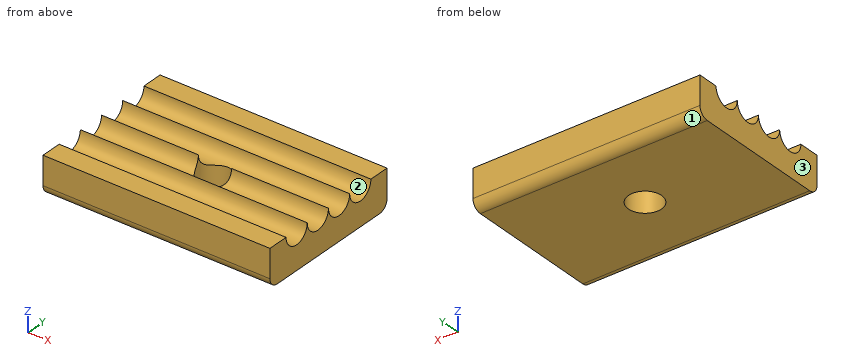
from build123d import *

# Parameters (mm, degrees)
SKETCH2_W           = 24
SKETCH2_H           = 16
BOSS_EXTRUDE1_DEPTH = 4
SKETCH3_R           = 1.75
CUT_EXTRUDE1_DEPTH  = 5
FILLET1_R           = 1
CUT_EXTRUDE2_DEPTH  = 29


with BuildPart() as part:
    # Sketch2 → Boss-Extrude1 (new body)
    with BuildSketch(Plane.XY):
        with Locations((6.957345972, -4)):
            Rectangle(SKETCH2_W, SKETCH2_H)
    extrude(amount=BOSS_EXTRUDE1_DEPTH)

    # Sketch3 → Cut-Extrude1 (cut)
    with BuildSketch(Plane.XY.offset(4)):
        with Locations((6.957345972, -4)):
            Circle(SKETCH3_R)
    extrude(amount=-CUT_EXTRUDE1_DEPTH, mode=Mode.SUBTRACT)

    # Fillet1
    fillet1_edges = [part.edges().sort_by_distance(p)[0] for p in [
        (6.957345972, 4, 0),
        (6.957345972, -12, 0),
    ]]
    fillet(fillet1_edges, radius=FILLET1_R)

    # Sketch4 → Cut-Extrude2 (cut)
    with BuildSketch(Plane.ZY.offset(5.042654028)):
        with BuildLine():
            ThreePointArc((5.45, -8.35), (5.025304833, -7.324695167), (4, -6.9))
            Line((4, -6.9), (4, -9.8))
            ThreePointArc((4, -9.8), (5.025304833, -9.375304833), (5.45, -8.35))
        make_face()
        with BuildLine():
            Line((4, -9.8), (4, -6.9))
            ThreePointArc((4, -6.9), (2.55, -8.35), (4, -9.8))
        make_face()
        with BuildLine():
            ThreePointArc((4, -6.9), (5.025304833, -6.475304833), (5.45, -5.45))
            ThreePointArc((5.45, -5.45), (5.025304832, -4.424695167), (3.999999999, -4))
            Line((4, -4), (4, -6.9))
        make_face()
        with BuildLine():
            Line((4, -6.9), (4, -4))
            ThreePointArc((3.999999999, -4), (2.55, -5.450000001), (4, -6.9))
        make_face()
        with BuildLine():
            ThreePointArc((4, -1.1), (2.55, -2.549999999), (3.999999999, -4))
            Line((4, -4), (4, -1.1))
        make_face()
        with BuildLine():
            Line((4, -1.1), (4, -4))
            ThreePointArc((3.999999999, -4), (5.025304832, -3.575304833), (5.45, -2.55))
            ThreePointArc((5.45, -2.55), (5.025304833, -1.524695167), (4, -1.1))
        make_face()
        with BuildLine():
            ThreePointArc((4, 1.8), (2.55, 0.35), (4, -1.1))
            Line((4, -1.1), (4, 1.8))
        make_face()
        with BuildLine():
            Line((4, 1.8), (4, -1.1))
            ThreePointArc((4, -1.1), (5.025304833, -0.675304833), (5.45, 0.35))
            ThreePointArc((5.45, 0.35), (5.025304833, 1.375304833), (4, 1.8))
        make_face()
    extrude(amount=-CUT_EXTRUDE2_DEPTH, mode=Mode.SUBTRACT)


solid = part.part
Build history of the part. All positions in model axes, mm. Face numbers are marked on the shaded views. Coordinates: 2 decimals unless noted, no trailing zeros. Order: outer loops, then holes, each group sorted by start corner. A loop starts at its lowest first (then second) coordinate and runs counter-clockwise, first axis right, second up. Notation, with made-up numbers: (82, 5.25) - (113, 5.25) arc R23 cw to (113, 44.25) - close; hole circle Ø7 at (36.5, -13.75). An arc over 180 degrees is marked (long way). Write item = value, one per line. Start each with the question number.
1) Flat gauge pin, fed straight in: pin 1 Ø3 at (x, y) = (6.96, -4) entering from +Z. Where does the tip first touch, or does it go through?
2) Saw through at C-C on y = -5.45. Write the cut outline in (x, z), then the cut area to 3 significant figures.
3) Saw through at B-B on x = 2. Write the cut outline in (y, z).
4) Wall check: line 1 along X through (y, z) = (-4, 0.9); line 2 along Y through (x, z) = (15.5, 3.5); line 3 along Y through (x, z) = (-0.75, 2.7). Give the ranges that are in metal, low to high. Write a range as from..to.
5) Saw through at A-A on z = 3. Write the cut outline in (x, y).
6) Two-plate mould, pull along Y, no slides. Class the marked faces 1, 2 and 3: pulls with the +Y half, pulls with the -Y half, needs draft (parallel to the pull), parting line crosses it, or undercut.
7) Saw through at D-D on z = 1.8. Write the cut outline in (x, y).
From the geometry:
q1.pin_1 = through
q2.outline = (-5.04, 0) - (5.98, 0) - (5.98, 2.55) - (-5.04, 2.55) - close; (7.94, 0) - (18.96, 0) - (18.96, 2.55) - (7.94, 2.55) - close
q2.area = 56.2 mm^2
q3.outline = (-12, 1) arc R1 ccw to (-11, 0) - (3, 0) arc R1 ccw to (4, 1) - (4, 4) - (1.8, 4) arc R1.45 cw to (-1.1, 4) arc R1.45 cw to (-4, 4) arc R1.45 cw to (-6.9, 4) arc R1.45 cw to (-9.8, 4) - (-12, 4) - close
q4.line_1 = -5.04..5.21, 8.71..18.96
q4.line_2 = -12..-9.71, -6.99..-6.81, -4.09..-3.91, -1.19..-1.01, 1.71..4
q4.line_3 = -12..-8.99, -7.71..-6.09, -4.81..-3.19, -1.91..-0.29, 0.99..4
q5.outline = (-5.04, -12) - (18.96, -12) - (18.96, -9.4) - (-5.04, -9.4) - close; (-5.04, -7.3) - (18.96, -7.3) - (18.96, -6.5) - (-5.04, -6.5) - close; (-5.04, -4.4) - (5.25, -4.4) arc R1.75 cw to (5.25, -3.6) - (-5.04, -3.6) - close; (-5.04, -1.5) - (18.96, -1.5) - (18.96, -0.7) - (-5.04, -0.7) - close; (-5.04, 1.4) - (18.96, 1.4) - (18.96, 4) - (-5.04, 4) - close; (8.66, -4.4) - (18.96, -4.4) - (18.96, -3.6) - (8.66, -3.6) arc R1.75 cw to start
q6.face_1 = pulls with the +Y half
q6.face_2 = undercut
q6.face_3 = needs draft
q7.outline = (-5.04, -12) - (18.96, -12) - (18.96, 4) - (-5.04, 4) - close; hole circle Ø3.5 at (6.96, -4)
